Can you work these out from the drawing? Everything is in mm from the part's minimum corner. A direction names the side the tool comes from. Give positions to 0.01 mm unless a question says otherwise; leave off trailing zeros. Loops run counter-clockwise (first coordinate to the right, second up) from the corner with the lowest first, then second, coordinate; pieces in that order, holes last. Notation, with made-up numbers: M 17.5,-35.75 L 45.5,-35.75 A22 ccw 45.5,-10.75 Z; hole C -24.5,54 d5. An arc over 180 degrees is marked long. Use CSV: the item, a comma, the result in double quotes.
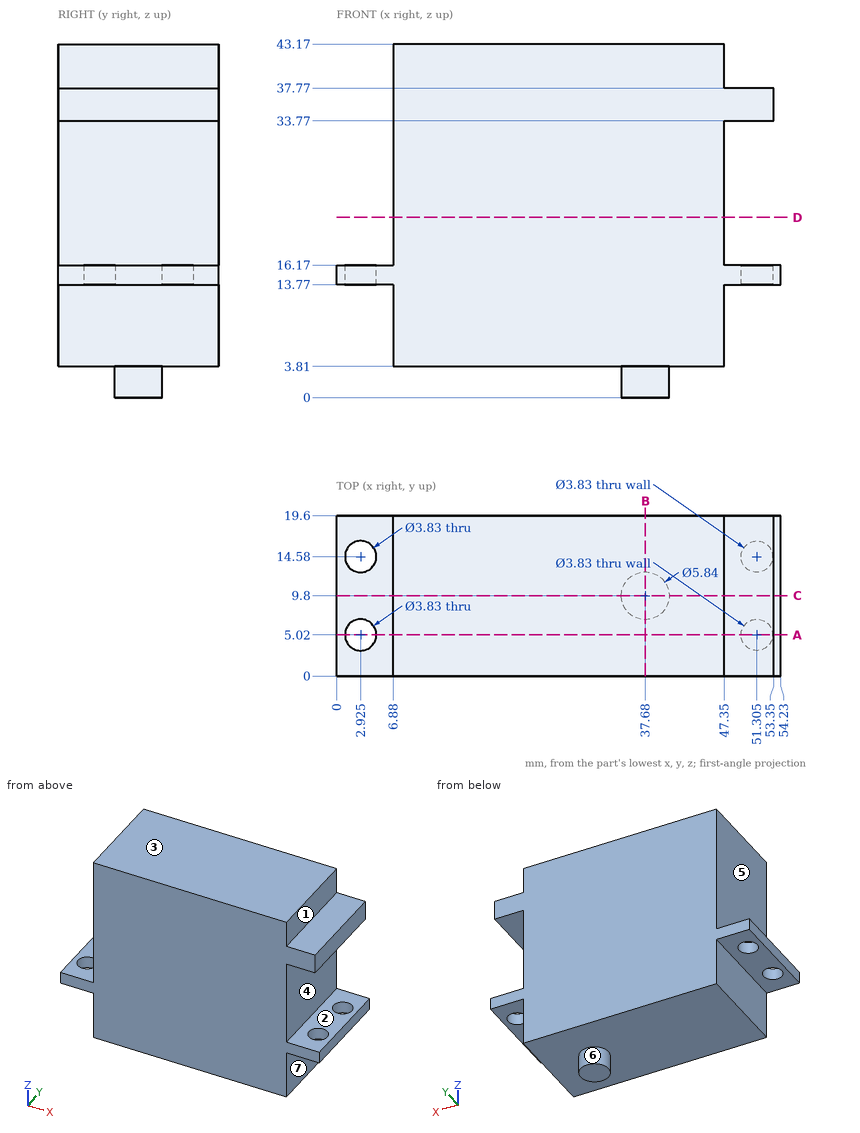
Q1. If we mould it in two halves opening along Z, with no side actions, what happens to the marked faces 1, 2 and 3? For each: released by +Z, released by -Z, zero draft, split by the parting line, or undercut.
Model answer:
face 1,"zero draft"
face 2,"undercut"
face 3,"released by +Z"
Q2. I want a section at D-D, the plane z = 22. Please give me the cut outline in (x, y), then the cut area to 3 significant figures.
Model answer:
outline,"M 6.88,0 L 47.35,0 L 47.35,19.6 L 6.88,19.6 Z"
area,"793 mm2"
Q3. I want a section at B-B, the plane x = 37.68. Please give me the cut outline in (y, z).
Model answer:
outline,"M 0,3.81 L 6.88,3.81 L 6.88,0 L 12.72,0 L 12.72,3.81 L 19.6,3.81 L 19.6,43.17 L 0,43.17 Z"
Q4. For the marked faces 4, 5, 6 and 7, which set-ups out of +Z, -Z, +X, -X, +Y, -Y let a thin tool reach every point of the face, with its end or its side?
Model answer:
face 4,"+X, +Y, -Y"
face 5,"+Z, -X, +Y, -Y"
face 6,"-Z"
face 7,"-Z, +X, +Y, -Y"
Q5. I'm going to push flat-ended pins straight in: P1, Ø10, axis at x = 26, y = 8, coming from the -Z side; P2, Ø4.5, axis at x = 51.305, y = 14.58, coming from the -Z side; P3, Ø1.2, axis at y = 9.5, z = 36, coming from the +X side; P4, Ø2.5, axis at x = 2.925, y = 14.58, coming from the -Z side. Where does each tip first touch, or does it pass through?
Model answer:
P1,"z = 3.81"
P2,"z = 13.77"
P3,"x = 53.35"
P4,"through"
Q6. I want a section at A-A, the plane y = 5.02. Please give me the cut outline in (x, z).
Model answer:
outline,"M 0,13.77 L 1.01,13.77 L 1.01,16.17 L 0,16.17 Z; M 4.84,13.77 L 6.88,13.77 L 6.88,3.81 L 47.35,3.81 L 47.35,13.77 L 49.39,13.77 L 49.39,16.17 L 47.35,16.17 L 47.35,33.77 L 53.35,33.77 L 53.35,37.77 L 47.35,37.77 L 47.35,43.17 L 6.88,43.17 L 6.88,16.17 L 4.84,16.17 Z; M 53.22,13.77 L 54.23,13.77 L 54.23,16.17 L 53.22,16.17 Z"
Q7. Please list where these lines run through material, in increasing order: L1, parallel to Z at x = 47.5, y = 17.5; L2, parallel to Z at x = 26, y = 5.25; L3, parallel to X at y = 14.25, z = 39. Write a range as from..to.
Model answer:
L1,"13.77..16.17, 33.77..37.77"
L2,"3.81..43.17"
L3,"6.88..47.35"
Q8. I want a section at C-C, the plane y = 9.8. Please give me the cut outline in (x, z).
Model answer:
outline,"M 0,13.77 L 6.88,13.77 L 6.88,3.81 L 34.76,3.81 L 34.76,0 L 40.6,0 L 40.6,3.81 L 47.35,3.81 L 47.35,13.77 L 54.23,13.77 L 54.23,16.17 L 47.35,16.17 L 47.35,33.77 L 53.35,33.77 L 53.35,37.77 L 47.35,37.77 L 47.35,43.17 L 6.88,43.17 L 6.88,16.17 L 0,16.17 Z"
